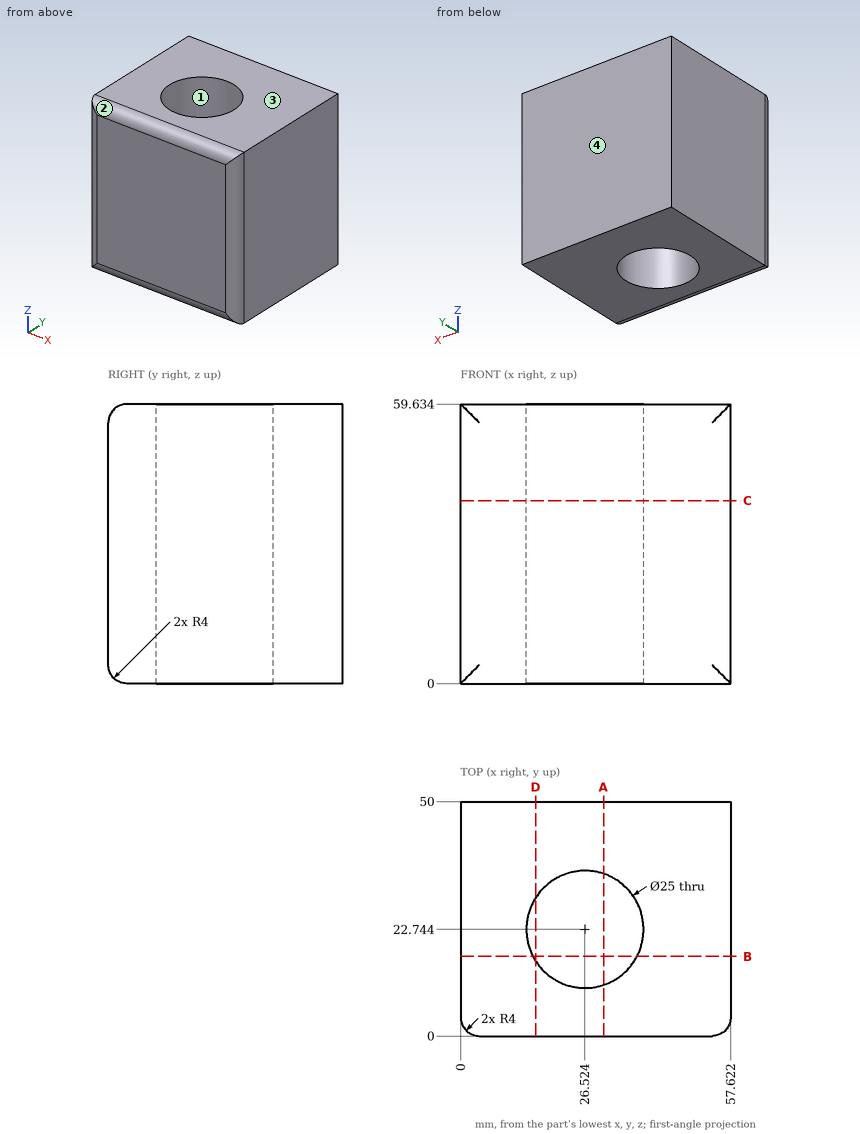
Print and shaded views of the part. All mm, measured from the part's lowest x, y and z. Coordinates: 2 decimals unless noted, no trailing zeros. Loops run counter-clockwise (first coordinate to the right, second up) from the corner with the lowest first, then second, coordinate; pieces in that order, holes last. Notation, with made-up numbers: (14, -6) -> (65, -6) arc R23 ccw to (65, 18) -> close; hole circle Ø10 at (57.25, 0). An arc over 180 degrees is marked (long way). Use a Markdown table: item, result. Add a question column.
Item 1: Pull direction Y, two halves, no side cores. Call the marked faces 1, 2, 3 and 4: +Y half, -Y half, draft (parallel to the pull), parting line (faces both ways), or undercut.
Item 2: Band-saw the part on A-A on x = 30.5. Write the cut outline in (y, z) (1 decimal), plus the area to 3 significant figures.
Item 3: Band-saw the part on D-D on x = 16. Write the cut outline in (y, z).
Item 4: Band-saw the part on C-C on z = 39. Write the cut outline in (x, y) (1 decimal).
Item 5: Band-saw the part on B-B on y = 17. Write the cut outline in (x, z).
Item 6: Probe probe 1 along Y at (x, z) = (29.5, 30) (1 decimal); probe 2 along X at (y, z) = (18.5, 27); probe 3 along Y at (x, z) = (28.5, 13.5). List the from-to ranges inside material, lowest first.
Geometry says:
| question | item | result |
|---|---|---|
| 1 | face 1 | undercut |
| 1 | face 2 | -Y half |
| 1 | face 3 | draft |
| 1 | face 4 | +Y half |
| 2 | outline | (0, 4) arc R4 ccw to (4, 0) -> (10.9, 0) -> (10.9, 59.6) -> (4, 59.6) arc R4 ccw to (0, 55.6) -> close; (34.6, 0) -> (50, 0) -> (50, 59.6) -> (34.6, 59.6) -> close |
| 2 | area | 1,560 mm² |
| 3 | outline | (0, 4) arc R4 ccw to (4, 0) -> (16, 0) -> (16, 59.63) -> (4, 59.63) arc R4 ccw to (0, 55.63) -> close; (29.49, 0) -> (50, 0) -> (50, 59.63) -> (29.49, 59.63) -> close |
| 4 | outline | (0, 4) arc R4 ccw to (4, 0) -> (53.6, 0) arc R4 ccw to (57.6, 4) -> (57.6, 50) -> (0, 50) -> close; hole circle Ø25 at (26.5, 22.7) |
| 5 | outline | (0, 0) -> (15.42, 0) -> (15.42, 59.63) -> (0, 59.63) -> close; (37.63, 0) -> (57.62, 0) -> (57.62, 59.63) -> (37.63, 59.63) -> close |
| 6 | probe 1 | 0 to 10.6, 34.9 to 50 |
| 6 | probe 2 | 0 to 14.77, 38.28 to 57.62 |
| 6 | probe 3 | 0 to 10.4, 35.09 to 50 |
